```python
from build123d import *

# Parameters (mm, degrees)
EXTRUDE1_DEPTH           = 63.5
F_10_CLEARANCE_HOLE1_D   = 5.6134
F_7_16_CLEARANCE_HOLE1_D = 11.50874


with BuildPart() as part:
    # Sketch1 → Extrude1 (new body)
    with BuildSketch(Plane.XY):
        with BuildLine():
            Line((0, 0), (0, 38.1))
            Line((0, 38.1), (1.5875, 38.1))
            ThreePointArc((1.5875, 38.1), (3.83256403, 37.17006403), (4.7625, 34.925))
            Line((4.7625, 34.925), (4.7625, 9.525))
            ThreePointArc((4.7625, 9.525), (6.157403955, 6.157403955), (9.525, 4.7625))
            Line((9.525, 4.7625), (34.925, 4.7625))
            ThreePointArc((34.925, 4.7625), (37.17006403, 3.83256403), (38.1, 1.5875))
            Line((38.1, 1.5875), (38.1, 0))
            Line((38.1, 0), (0, 0))
        make_face()
    extrude(amount=EXTRUDE1_DEPTH)

    # #10 Clearance Hole1 (through all)
    with Locations(Plane(origin=(0, 4.7625, 0), x_dir=(-1, 0, 0), z_dir=(0, 1, 0))):
        with Locations((-19.05, 50.8), (-19.05, 12.7)):
            Hole(F_10_CLEARANCE_HOLE1_D / 2)

    # 7/16 Clearance Hole1 (through all)
    with Locations(Plane(origin=(4.7625, 0, 0), x_dir=(0, 0, -1), z_dir=(1, 0, 0))):
        with Locations((-31.75, 25.4)):
            Hole(F_7_16_CLEARANCE_HOLE1_D / 2)


solid = part.part
```
Geometry: final body of the model. Coordinates: model frame, mm. A direction names the side the tool comes from. Round coordinates to 2 decimals unless told otherwise and drop trailing zeros. Order: outer loops, then holes, each group sorted by start corner. A loop starts at its lowest first (then second) coordinate and runs counter-clockwise, first axis right, second up. Notation, with made-up numbers: (30, 64.5) -> (88, 64.5) arc R24 ccw to (88, 82.5) -> close; hole circle Ø5 at (77.25, 41.5). An arc over 180 degrees is marked (long way). Use CSV: the item, a comma, the result in double quotes. Start each with the question number.
1) Set-up query: faces 1 (the face through (0, 19, 31)), 2 (the face through (4.762, 17, 31)). Return all of +Z, -Z, +X, -X, +Y, -Y with unobstructed straight access to the full face (end or side cutting, diameter ignored); none if empty.
2) Draft query along Z for faces 3 (the face through (2.348, 19.782, 30.503)), 4 (the face through (19, 0, 31)), 5 (the face through (12, 4, 0)). Return one class per face: +Z half, -Z half, draft (parallel to the pull), parting line (faces both ways), or undercut.
3) First-contact query: pin 1 Ø6 at (y, z) = (30.5, 44.5) entering from +X; pin 2 Ø1 at (x, z) = (25.5, 49) entering from -Y; pin 3 Ø12 at (x, z) = (18, 8.5) entering from +Y. Flat tips, straight axial feed; report the tip coordinate or a pass-through.
4) Section C-C (y = 25.4). Return the cut outline in (x, z).
5) Section B-B (x = 19.05). Return the cut outline in (y, z), and give its area (3 significant figures).
6) Material intervals for line 1 along Z through (x, y) = (19, 3); line 2 along Y through (x, z) = (1.6, 31.75); line 3 along Y through (x, z) = (29.5, 26.5), sorted ascending. Write a range as from..to.
Returned:
1,face 1,"+Z, -Z, -X, +Y, -Y"
1,face 2,"+Z, -Z, +X, +Y"
2,face 3,"undercut"
2,face 4,"draft"
2,face 5,"-Z half"
3,pin 1,"stops at x = 4.76"
3,pin 2,"stops at y = 0"
3,pin 3,"stops at y = 4.76"
4,outline,"(0, 0) -> (4.76, 0) -> (4.76, 26) -> (0, 26) -> close; (0, 37.5) -> (4.76, 37.5) -> (4.76, 63.5) -> (0, 63.5) -> close"
5,outline,"(0, 0) -> (4.76, 0) -> (4.76, 9.89) -> (0, 9.89) -> close; (0, 15.51) -> (4.76, 15.51) -> (4.76, 47.99) -> (0, 47.99) -> close; (0, 53.61) -> (4.76, 53.61) -> (4.76, 63.5) -> (0, 63.5) -> close"
5,area,"249 mm²"
6,line 1,"z = 0..9.89, 15.51..47.99, 53.61..63.5"
6,line 2,"y = 0..19.65, 31.15..38.1"
6,line 3,"y = 0..4.76"
